from build123d import *

# Parameters (mm, degrees)
F0_R     = 38.1
F1_DEPTH = 76.2
F2_DEPTH = 23.8125
F3_DEPTH = 63.5


with BuildPart() as f1:
    # F0 (on Top) → F1 (new body)
    with BuildSketch(Plane.XY):
        with BuildLine():
            ThreePointArc((49.1259336968, -12.9337789688), (50.3797450956, -6.5208346169), (50.8, 0))
            ThreePointArc((50.8, 0), (50.3797450956, 6.5208346169), (49.1259336968, 12.9337789688))
            ThreePointArc((49.1259336968, 12.9337789688), (0, 50.8), (-49.1259336968, 12.9337789688))
            ThreePointArc((-49.1259336968, 12.9337789688), (-50.8, 0), (-49.1259336968, -12.9337789688))
            ThreePointArc((-49.1259336968, -12.9337789688), (0, -50.8), (49.1259336968, -12.9337789688))
        make_face()
        Circle(F0_R, mode=Mode.SUBTRACT)
        Circle(F0_R)
    extrude(amount=F1_DEPTH)

    # F0 (on Top) → F2 (join)
    with BuildSketch(Plane.XY):
        with BuildLine():
            ThreePointArc((-49.1259336968, -12.9337789688), (-50.8, 0), (-49.1259336968, 12.9337789688))
            Line((-49.1259336968, 12.9337789688), (-52.1963045529, 13.7421401544))
            ThreePointArc((-52.1963045529, 13.7421401544), (-53.975, 0), (-52.1963045529, -13.7421401544))
            Line((-52.1963045529, -13.7421401544), (-49.1259336968, -12.9337789688))
        make_face()
        with BuildLine():
            ThreePointArc((49.1259336968, 12.9337789688), (50.3797450956, 6.5208346169), (50.8, 0))
            ThreePointArc((50.8, 0), (50.3797450956, -6.5208346169), (49.1259336968, -12.9337789688))
            Line((49.1259336968, -12.9337789688), (52.1963045529, -13.7421401544))
            ThreePointArc((52.1963045529, -13.7421401544), (53.975, 0), (52.1963045529, 13.7421401544))
            Line((52.1963045529, 13.7421401544), (49.1259336968, 12.9337789688))
        make_face()
    extrude(amount=F2_DEPTH)

    # F0 (on Top) → F3 (cut)
    with BuildSketch(Plane.XY):
        Circle(F0_R)
    extrude(amount=F3_DEPTH, mode=Mode.SUBTRACT)


solid = f1.part
Input: part model. Units: mm. Frame: model coordinates. A direction names the side the tool comes from. Give positions to 0.01 mm unless a question says otherwise; leave off trailing zeros. Order: outer loops, then holes, each group sorted by start corner. A loop starts at its lowest first (then second) coordinate and runs counter-clockwise, first axis right, second up. Notation, with made-up numbers: M 82,-33 L 121,-33 A24 cw 121,3 Z; hole C 50,84 d1. An arc over 180 degrees is marked long. Answer as a JSON object with one key per item and string values.
1. Ray query, line 1 (Z direction, x = 1, y = -19.5); line 2 (Y direction, x = 6, z = 25); line 3 (X direction, y = -27, z = 49). Return the intervals inside material, ascending. Write a range as [from, to].
Result sheet:
{"line 1": "[63.5, 76.2]", "line 2": "[-50.44, -37.62], [37.62, 50.44]", "line 3": "[-43.03, -26.88], [26.88, 43.03]"}
2. Pull-direction query (X, two-part tool) for faces 4 (the cylindrical face through (-53.975, 0.195, 11.74)), 5 (the cylindrical face through (53.975, -0.195, 11.74)), 6 (the flat face through (50.683, 13.344, 11.74)); classes: +X half, -X half, draft (parallel to the pull), parting line (faces both ways), or undercut.
Result sheet:
{"face 4": "-X half", "face 5": "+X half", "face 6": "undercut"}
3. Cut plane C-C, the plane y = 30. Output: boundary loops of the cut face in (x, z), and give its area (3 significant figures).
Result sheet:
{"outline": "M -41,0 L -23.49,0 L -23.49,63.5 L 23.49,63.5 L 23.49,0 L 41,0 L 41,76.2 L -41,76.2 Z", "area": "3,260 mm²"}
4. Cut plane D-D, the plane y = -6. Output: boundary loops of the cut face in (x, z), and give its area (3 significant figures).
Result sheet:
{"outline": "M -53.64,0 L -37.62,0 L -37.62,63.5 L 37.62,63.5 L 37.62,0 L 53.64,0 L 53.64,23.81 L 50.44,23.81 L 50.44,76.2 L -50.44,76.2 L -50.44,23.81 L -53.64,23.81 Z", "area": "3,060 mm²"}
5. Cut plane B-B, the plane z = 27.5. Output: boundary loops of the cut face in (x, y), and give its area (3 significant figures).
Result sheet:
{"outline": "C 0,0 d101.6; hole C 0,0 d76.2", "area": "3,550 mm²"}
6. Cut plane A-A, the plane x = 0. Output: boundary loops of the cut face in (y, z), and give its area (3 significant figures).
Result sheet:
{"outline": "M -50.8,0 L -38.1,0 L -38.1,63.5 L 38.1,63.5 L 38.1,0 L 50.8,0 L 50.8,76.2 L -50.8,76.2 Z", "area": "2,900 mm²"}
7. Reachability of faces 1 (the flat face through (50.64, -13.332, 11.74)), 2 (the flat face through (-50.64, 13.332, 11.74)), 3 (the cylindrical face through (-30.235, -23.183, 31.306)) from +Z, -Z, +X, -X, +Y, -Y: full face, straight path, thin tool, end or side. Return the list, or none.
Result sheet:
{"face 1": "+Z, -Z, -Y", "face 2": "+Z, -Z, +Y", "face 3": "-Z"}
8. First-contact query: P1, Ø8, axis at x = -36.5, z = 13, coming from the -Y side; P2, Ø2, axis at y = -34, z = 34, coming from the +X side; P3, Ø10, axis at y = -29, z = 40.5, coming from the +X side. Flat tips, straight axial feed; report the tip coordinate or a pass-through.
Result sheet:
{"P1": "y = -39.04", "P2": "x = 38.62", "P3": "x = 44.77"}
